CAD build for the part. Positions are in the model's coordinates, mm. A direction names the side the tool comes from. Give positions to 0.01 mm unless a question says otherwise; leave off trailing zeros. Order: outer loops, then holes, each group sorted by start corner. A loop starts at its lowest first (then second) coordinate and runs counter-clockwise, first axis right, second up.
Item 1: Band-saw the part on C-C on z = 7. Give the cut face in (x, y).
Item 2: Band-saw the part on A-A on y = -6. Give the cut face in (x, z), plus the area to 3 significant figures.
Item 3: Band-saw the part on D-D on z = 4.75. Count the separate pieces of the cut face and the enclosed holes in it, plus the area to 3 significant figures.
Item 4: Two-plate mould, pull along Y, no slides. Class faces 4 (the flat face through (14, 8.85, 8)), 5 (the cylindrical face through (5.89, -5.2, 5.32)), 6 (the flat face through (14, -8.85, 8)), 7 (the cylindrical face through (-5.5, 6.1, 5.3)): released by +Y, released by -Y, zero draft, split by the parting line, or undercut.
Item 5: Wall check: L1, parallel to Y at x = 12.5, z = 1.5; L2, parallel to Y at x = 6.5, z = 3.5. Give the ranges that are in metal, low to high.
Item 6: Band-saw the part on B-B on x = 6.5. Give the cut face in (y, z), plus the area to 3 significant figures.
Item 7: Which spindle directions (+Z, -Z, +X, -X, +Y, -Y) get a long thin tool onto all of the face, cutting with end or side? Do faces 1 (the flat face through (0, 0, 10)), 2 (the flat face through (8.85, 14, 8)), 3 (the flat face through (8.85, -14, 8)). Say none if no direction does.
Item 8: Flat gauge pins, fed straight in: P1, Ø2, axis at x = 11.5, y = -11, coming from the +Z side; P2, Ø2.5, axis at x = 12.5, y = -12.5, coming from the +Z side; P3, Ø0.9, axis at x = 14.5, z = 9, coming from the -Y side; P4, Ø1.5, axis at y = 13.5, z = 9, coming from the +X side. Where does each tip first touch, or does it go through?
Solid Edge part; units mm, degrees
sketch "Sketch1" plane through (0, 0, 0) normal (0, 0, 1) x (1, 0, 0)
  line L0 (-15.5, -15.5) -> (15.5, -15.5)
  line L1 (15.5, -15.5) -> (15.5, 15.5)
  line L2 (15.5, 15.5) -> (-15.5, 15.5)
  line L3 (-15.5, 15.5) -> (-15.5, -15.5)
  circle A0 centre (-12.5, -12.5) radius 2.1
  circle A1 centre (-12.5, 12.5) radius 2.1
  circle A2 centre (12.5, 12.5) radius 2.1
  circle A3 centre (12.5, -12.5) radius 2.1
  dimension "D1" = 15.5
  dimension "D2" = 15.5
extrude "Protrusion1" add sketch "Sketch1" along normal blind 10.5
hole "Hole_1" at (-6.5, -6, 10.5) direction (0, 0, -1) diameter 2.013 end up to next
hole "Hole1" at (-6.5, 6, 10.5) direction (0, 0, -1) diameter 2.013 end up to next
hole "Hole2" at (6.5, 6, 10.5) direction (0, 0, -1) diameter 2.013 end up to next
hole "Hole3" at (6.5, -6, 10.5) direction (0, 0, -1) diameter 2.013 end up to next
sketch "Sketch2" plane through (0, 0, 10.5) normal (0, 0, 1) x (0, 1, 0)
  line L0 (-1.6, -15.5) -> (1.6, -15.5)
  line L1 (1.6, -15.5) -> (1.6, 15.5)
  line L2 (1.6, 15.5) -> (-1.6, 15.5)
  line L3 (-1.6, 15.5) -> (-1.6, -15.5)
  dimension "D1" = 1.6
extrude "ExtrudedCutout_1" cut sketch "Sketch2" against normal blind 0.5
sketch "Sketch3" plane through (0, -8.575, 10.5) normal (0, 0, 1) x (0, 1, 0)
  line L0 (-6.925, -8.85) -> (-3.925, -8.85)
  arc A0 (-3.925, -8.85) -> (-0.275, -12.5) centre (-3.925, -12.5) cw
  line L1 (-0.275, -15.5) -> (-0.275, -12.5)
  dimension "D1" = 0.275
  dimension "D2" = 6.925
extrude "ExtrudedCutout_2" cut sketch "Sketch3" against normal blind 4.1 material side at (8.9, -14, 10.5)
pattern_circular "Pattern2" count 4 over 360 about axis through (0, 0, 10.5) along (0, 0, -1) of "ExtrudedCutout_2"
The answers:
1. outline: (-15.5, -8.85) - (-12.5, -8.85) arc R3.65 cw to (-8.85, -12.5) - (-8.85, -15.5) - (8.85, -15.5) - (8.85, -12.5) arc R3.65 cw to (12.5, -8.85) - (15.5, -8.85) - (15.5, 8.85) - (12.5, 8.85) arc R3.65 cw to (8.85, 12.5) - (8.85, 15.5) - (-8.85, 15.5) - (-8.85, 12.5) arc R3.65 cw to (-12.5, 8.85) - (-15.5, 8.85) - close; hole circle Ø2.01 at (-6.5, -6); hole circle Ø2.01 at (-6.5, 6); hole circle Ø2.01 at (6.5, -6); hole circle Ø2.01 at (6.5, 6)
2. outline: (-15.5, 0) - (-7.51, 0) - (-7.51, 10.5) - (-15.5, 10.5) - close; (-5.49, 0) - (5.49, 0) - (5.49, 10.5) - (-5.49, 10.5) - close; (7.51, 0) - (15.5, 0) - (15.5, 10.5) - (7.51, 10.5) - close
2. area: 283 mm2
3. separate pieces: 1
3. enclosed holes: 8
3. area: 893 mm2
4. face 4: released by +Y
4. face 5: undercut
4. face 6: released by -Y
4. face 7: undercut
5. L1: y = -15.5 to -14.6, -10.4 to 10.4, 14.6 to 15.5
5. L2: y = -15.5 to -7.01, -4.99 to 4.99, 7.01 to 15.5
6. outline: (-15.5, 0) - (-7.01, 0) - (-7.01, 10.5) - (-15.5, 10.5) - close; (-4.99, 0) - (4.99, 0) - (4.99, 10.5) - (1.6, 10.5) - (1.6, 10) - (-1.6, 10) - (-1.6, 10.5) - (-4.99, 10.5) - close; (7.01, 0) - (15.5, 0) - (15.5, 10.5) - (7.01, 10.5) - close
6. area: 282 mm2
7. face 1: +Z, +X, -X
7. face 2: +Z, +X, +Y
7. face 3: +Z, +X, -Y
8. P1: stops at z = 6.4
8. P2: passes through
8. P3: stops at y = -8.85
8. P4: stops at x = 8.85
